from build123d import *

# Parameters (mm, degrees)
SKETCH1_W                     = 6
SKETCH1_H                     = 21
BOSS_EXTRUDE1_DEPTH           = 104
SKETCH2_W                     = 35.5
SKETCH2_H                     = 1.5
CUT_EXTRUDE1_DEPTH            = 119.61729427
CBORE_FOR_M3_SHCS1_AT_2_COUNT = 2
CBORE_FOR_M3_SHCS1_AT_2_PITCH = 20
CBORE_FOR_M3_SHCS2_AT_2_COUNT = 2
CBORE_FOR_M3_SHCS2_AT_2_PITCH = 58
CBORE_FOR_M3_SHCS2_AT_3_COUNT = 2
CBORE_FOR_M3_SHCS2_AT_3_PITCH = 78.811735167
CBORE_FOR_M3_SHCS2_AT_4_COUNT = 2
CBORE_FOR_M3_SHCS2_AT_4_PITCH = 53.36
M3_CLEARANCE_HOLE1_D          = 3.4
SKETCH25_R                    = 2.165
CUT_EXTRUDE7_DEPTH            = 5
CUT_EXTRUDE8_START            = -5
SKETCH26_R                    = 2.165
CUT_EXTRUDE8_DEPTH            = 5
SKETCH28_W                    = 15
SKETCH28_H                    = 7
CUT_EXTRUDE10_DEPTH           = 1.5
FILLET3_R                     = 15
FILLET2_R                     = 3
CHAMFER1_SIZE                 = 1
CHAMFER2_SIZE                 = 0.4


with BuildPart() as part:
    # Sketch1 → Boss-Extrude1 (new body)
    with BuildSketch(Plane.XY):
        with Locations((-48.75, 13.5)):
            Rectangle(SKETCH1_W, SKETCH1_H)
        Polygon((-45.75, 3), (-51.75, 3), (-51.75, -3), (51.75, -3), (51.75, 3), (45.75, 3), align=None)
        with Locations((48.75, 13.5)):
            Rectangle(SKETCH1_W, SKETCH1_H)
    extrude(amount=-BOSS_EXTRUDE1_DEPTH)

    # Sketch2 → Cut-Extrude1 (cut, through all)
    with BuildSketch(Plane.XY):
        with Locations((0, 2.25)):
            Rectangle(SKETCH2_W, SKETCH2_H)
    extrude(amount=-CUT_EXTRUDE1_DEPTH, mode=Mode.SUBTRACT)

    # Sketch7 → CBORE for M3 SHCS1 (revolve, cut)
    with BuildSketch(Plane(origin=(-10, -3, -30), x_dir=(0, 0, -1), z_dir=(1, 0, 0))):
        Polygon((0, 0), (0, 4.5), (2.2, 4.5), (1.7, 4), (1.7, 3.5), (2.2, 3), (3.25, 3), (3.25, 0.5), (3.75, 0), align=None)
    cbore_for_m3_shcs1 = revolve(axis=Axis((-10, -9.35, -30), (0, 1, 0)), mode=Mode.SUBTRACT)

    # CBORE for M3 SHCS1 at 2: CBORE for M3 SHCS1 ×2
    with Locations(*[(i * CBORE_FOR_M3_SHCS1_AT_2_PITCH, 0, 0) for i in range(1, CBORE_FOR_M3_SHCS1_AT_2_COUNT)]):
        add(cbore_for_m3_shcs1, mode=Mode.SUBTRACT)

    # Sketch19 → CBORE for M3 SHCS2 (revolve, cut)
    with BuildSketch(Plane(origin=(-29, 3, -25.32), x_dir=(0, 0, 1), z_dir=(1, 0, 0))):
        Polygon((0, 0), (0, 6), (2.2, 6), (1.7, 5.5), (1.7, 3.5), (2.2, 3), (3.25, 3), (3.25, 0.5), (3.75, 0), align=None)
    cbore_for_m3_shcs2 = revolve(axis=Axis((-29, 9.35, -25.32), (0, -1, 0)), mode=Mode.SUBTRACT)

    # CBORE for M3 SHCS2 at 2: CBORE for M3 SHCS2 ×2
    with Locations(*[(i * CBORE_FOR_M3_SHCS2_AT_2_PITCH, 0, 0) for i in range(1, CBORE_FOR_M3_SHCS2_AT_2_COUNT)]):
        add(cbore_for_m3_shcs2, mode=Mode.SUBTRACT)

    # CBORE for M3 SHCS2 at 3: CBORE for M3 SHCS2 ×2
    with Locations(*[Vector(0.7359310117618296, 0, -0.6770565308208834) * (i * CBORE_FOR_M3_SHCS2_AT_3_PITCH) for i in range(1, CBORE_FOR_M3_SHCS2_AT_3_COUNT)]):
        add(cbore_for_m3_shcs2, mode=Mode.SUBTRACT)

    # CBORE for M3 SHCS2 at 4: CBORE for M3 SHCS2 ×2
    with Locations(*[(0, 0, -i * CBORE_FOR_M3_SHCS2_AT_4_PITCH) for i in range(1, CBORE_FOR_M3_SHCS2_AT_4_COUNT)]):
        add(cbore_for_m3_shcs2, mode=Mode.SUBTRACT)

    # M3 Clearance Hole1 (through all)
    with Locations(Plane.ZY.offset(51.75)):
        with Locations((-96, 18), (-8, 18)):
            Hole(M3_CLEARANCE_HOLE1_D / 2)

    # Sketch25 → Cut-Extrude7 (cut)
    with BuildSketch(Plane.ZY.offset(51.75)):
        with Locations((-96, 18)):
            Circle(SKETCH25_R)
        with Locations((-8, 18)):
            Circle(SKETCH25_R)
    extrude(amount=-CUT_EXTRUDE7_DEPTH, mode=Mode.SUBTRACT)

    # Sketch26 → Cut-Extrude8 (cut)
    with BuildSketch(Plane(origin=(51.75, 0, 0), x_dir=(0, 0, -1), z_dir=(1, 0, 0)).offset(CUT_EXTRUDE8_START)):
        with Locations(Location((8, 18, 0), (0, 0, 180))):
            Circle(SKETCH26_R)
        with Locations(Location((96, 18, 0), (0, 0, 180))):
            Circle(SKETCH26_R)
    extrude(amount=CUT_EXTRUDE8_DEPTH, mode=Mode.SUBTRACT)

    # Sketch28 → Cut-Extrude10 (cut)
    with BuildSketch(Plane(origin=(0, 3, 0), x_dir=(1, 0, 0), z_dir=(0, 1, 0))):
        with Locations((-25.25, 3.5)):
            Rectangle(SKETCH28_W, SKETCH28_H)
        with Locations((25.25, 3.5)):
            Rectangle(SKETCH28_W, SKETCH28_H)
    extrude(amount=-CUT_EXTRUDE10_DEPTH, mode=Mode.SUBTRACT)

    # Fillet3
    fillet3_edges = [part.edges().sort_by_distance(p)[0] for p in [
        (17.75, 2.25, -7),
        (-17.75, 2.25, -7),
    ]]
    fillet(fillet3_edges, radius=FILLET3_R - 0.0001)  # a hair under: the kernel refuses the full size

    # Fillet2
    fillet2_edges = [part.edges().sort_by_distance(p)[0] for p in [
        (-51.75, 10.5, -104),
        (-32.75, 2.25, -7),
        (32.75, 2.25, -7),
        (51.75, 10.5, -104),
        (51.75, 10.5, 0),
        (-51.75, 10.5, 0),
    ]]
    fillet(fillet2_edges, radius=FILLET2_R)

    # Chamfer1
    chamfer1_edges = [part.edges().sort_by_distance(p)[0] for p in [
        (45.75, 3, -52),
        (-31.75, 3, -104),
        (47.25, 24, -104),
        (-47.25, 24, -104),
        (-47.25, 24, 0),
        (-51.75, 24, -52),
        (-50.871320344, 24, -0.878679656),
        (-50.871320344, 24, -103.121320344),
        (51.75, 24, -52),
        (47.25, 24, 0),
        (50.871320344, 24, -0.878679656),
        (50.871320344, 24, -103.121320344),
        (45.75, 13.5, -104),
        (31.75, 3, -104),
        (-45.75, 3, -52),
        (-45.75, 13.5, -104),
    ]]
    chamfer(chamfer1_edges, length=CHAMFER1_SIZE)

    # Chamfer2
    chamfer2_edges = [part.edges().sort_by_distance(p)[0] for p in [
        (-51.75, 18, -98.165),
        (-51.75, 18, -10.165),
        (51.75, 18, -10.165),
        (51.75, 18, -98.165),
    ]]
    chamfer(chamfer2_edges, length=CHAMFER2_SIZE)


solid = part.part
Check sheet for the modelled part. Datum: model origin and axes. Units: mm. A direction names the side the tool comes from. Give positions to 0.01 mm unless a question says otherwise; leave off trailing zeros. Write each loop counter-clockwise with the first axis right and the second up, starting at its lowest first coordinate (ties: lowest second). Pieces come first, ordered by that corner, then holes. Notation, with made-up numbers: (-13.75, 1.5) -> (23.25, 1.5) arc R25 cw to (23.25, 14.5) -> close; hole circle Ø4 at (86.25, 34). An arc over 180 degrees is marked (long way). Use one line per item in the form item = value. Start each with the question number.
1. Section check D-D (z = -96). Count the separate pieces of the cut face and the enclosed holes in it, and give its area (3 significant figures).
2. Access from +Z, -Z, +X, -X, +Y, -Y to the whole of each face (thin tool, end or side, straight path). Record for faces 4 (the cylindrical face through (49.018, 17.905, -98.163)), 5 (the cylindrical face through (-27.97, -1.49, -80.03)), 6 (the cylindrical face through (-49.082, 18.095, -98.163)), 7 (the cylindrical face through (-21.389, 2.24, -12.205)), 8 (the cylindrical face through (-25.827, 1.268, -79.385)).
3. Go/stop test with flat-tipped pins: P1, Ø5, axis at x = -28, z = -79, coming from the +Y side; P2, Ø2, axis at y = 18, z = -7.5, coming from the -X side; P3, Ø8, axis at x = 17.5, z = -64, coming from the +Y side; P4, Ø0.5, axis at y = 2, z = -1, coming from the +X side. Record where each tip stops, or that it passes through.
4. Section check B-B (y = 8). Record the cut outline in (x, z), and give its area (3 significant figures).
5. Mould release check, pull along Z, two halves, no side actions. Record for faces 1 (the flat face through (46.75, 20, -96)), 2 (the conical face through (50.453, 23.618, -1.334)), 3 (the cylindrical face through (-50.85, 9.82, -103.14)): pulls with the +Z half, pulls with the -Z half, needs draft (parallel to the pull), parting line crosses it, or undercut.
6. Section check C-C (z = -65). Record the cut outline in (x, y).
7. Thickness scan on line 1 along Z through (x, y) = (-29, 1); line 2 along Z through (x, y) = (-29, -1.9); line 3 along Y through (x, z) = (-50.35, -8) (3 decimals). Record the ranges inside material, lowest first. Write a range as from..to.
8. Section check A-A (x = 10). Record the cut outline in (y, z).
Conclusion:
q1.separate_pieces = 3
q1.enclosed_holes = 0
q1.area = 769 mm²
q2.face_4 = +X
q2.face_5 = +Y, -Y
q2.face_6 = -X
q2.face_7 = +Z, +Y
q2.face_8 = +Y
q3.P1 = 2.8
q3.P2 = through
q3.P3 = 3
q3.P4 = 51.19
q4.outline = (-51.75, -101) arc R3 ccw to (-48.75, -104) -> (-46.75, -104) -> (-45.75, -103) -> (-45.75, 0) -> (-48.75, 0) arc R3 ccw to (-51.75, -3) -> close; (45.75, -103) -> (46.75, -104) -> (48.75, -104) arc R3 ccw to (51.75, -101) -> (51.75, -3) arc R3 ccw to (48.75, 0) -> (45.75, 0) -> close
q4.area = 1,240 mm²
q5.face_1 = undercut
q5.face_2 = pulls with the +Z half
q5.face_3 = pulls with the -Z half
q6.outline = (-51.75, -3) -> (51.75, -3) -> (51.75, 23) -> (50.75, 24) -> (45.75, 24) -> (45.75, 4) -> (44.75, 3) -> (17.75, 3) -> (17.75, 1.5) -> (-17.75, 1.5) -> (-17.75, 3) -> (-44.75, 3) -> (-45.75, 4) -> (-45.75, 24) -> (-50.75, 24) -> (-51.75, 23) -> close
q7.line_1 = -104..-81.93, -75.43..-28.57, -22.07..0
q7.line_2 = -104..-80.38, -76.98..-27.02, -23.62..0
q7.line_3 = -3..15.835, 20.165..24
q8.outline = (-3, -104) -> (1.5, -104) -> (1.5, -32.2) -> (1, -31.7) -> (0.5, -31.7) -> (0, -32.2) -> (0, -33.25) -> (-2.5, -33.25) -> (-3, -33.75) -> close; (-3, -26.25) -> (-2.5, -26.75) -> (0, -26.75) -> (0, -27.8) -> (0.5, -28.3) -> (1, -28.3) -> (1.5, -27.8) -> (1.5, 0) -> (-3, 0) -> close
